Geometry: final body of the model. Coordinates: model frame, mm. Round coordinates to 2 decimals unless told otherwise and drop trailing zeros. Write each loop counter-clockwise with the first axis right and the second up, starting at its lowest first coordinate (ties: lowest second). Pieces come first, ordered by that corner, then holes. Notation, with made-up numbers: (27.25, 21) - (85.25, 21) arc R22 ccw to (85.25, 59) - close; hole circle Ø4 at (28.5, 14). An arc over 180 degrees is marked (long way). Use a Markdown table: item, result. Add a question column.
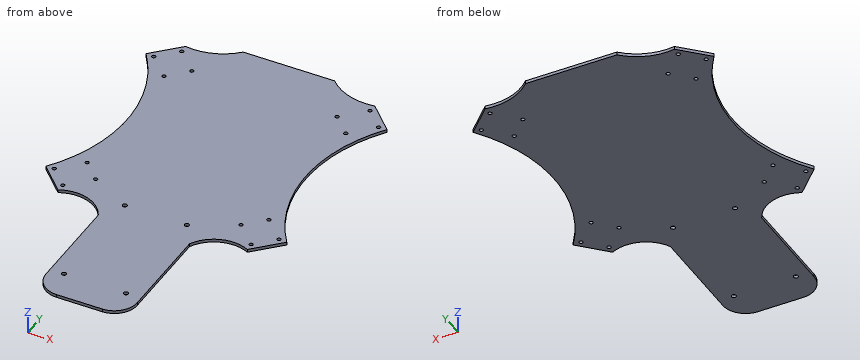
```python
from build123d import *

# Parameters (mm, degrees)
BOSS_EXTRUDE1_DEPTH = 2
SKETCH3_R           = 1.25
CUT_EXTRUDE1_DEPTH  = 188.552659272
SKETCH4_R           = 1.5
CUT_EXTRUDE2_DEPTH  = 188.552659272


with BuildPart() as part:
    # Sketch2 → Boss-Extrude1 (new body)
    with BuildSketch(Plane.XY):
        with BuildLine():
            Line((-79.195959493, 62.225396744), (-62.225396744, 79.195959493))
            ThreePointArc((-62.225396744, 79.195959493), (-44.806778225, 80.702789346), (-30, 90))
            Line((-30, 90), (30, 90))
            ThreePointArc((30, 90), (44.806778225, 80.702789346), (62.225396744, 79.195959493))
            Line((62.225396744, 79.195959493), (79.195959493, 62.225396744))
            ThreePointArc((79.195959493, 62.225396744), (58.781303002, 0), (79.195959493, -62.225396744))
            Line((79.195959493, -62.225396744), (62.225396744, -79.195959493))
            ThreePointArc((62.225396744, -79.195959493), (43.875108319, -77.923881554), (30, -90))
            Line((30, -90), (30, -155))
            ThreePointArc((30, -155), (25.606601718, -165.606601718), (15, -170))
            Line((15, -170), (-15, -170))
            ThreePointArc((-15, -170), (-25.606601718, -165.606601718), (-30, -155))
            Line((-30, -155), (-30, -90))
            ThreePointArc((-30, -90), (-43.875108319, -77.923881554), (-62.225396744, -79.195959493))
            Line((-62.225396744, -79.195959493), (-79.195959493, -62.225396744))
            ThreePointArc((-79.195959493, -62.225396744), (-58.781303002, 0), (-79.195959493, 62.225396744))
        make_face()
    extrude(amount=BOSS_EXTRUDE1_DEPTH)

    # Sketch3 → Cut-Extrude1 (cut, through all)
    with BuildSketch(Plane.XY.offset(2)):
        with Locations((-73.892658634, 61.871843354)):
            Circle(SKETCH3_R)
        with Locations((-59.75052301, 47.72970773)):
            Circle(SKETCH3_R)
        with Locations(Location((-61.871843354, 73.892658634, 0), (0, 0, 180))):
            Circle(SKETCH3_R)
        with Locations(Location((-47.72970773, 59.75052301, 0), (0, 0, 180))):
            Circle(SKETCH3_R)
        with Locations(Location((59.75052301, 47.72970773, 0), (0, 0, 180))):
            Circle(SKETCH3_R)
        with Locations(Location((73.892658634, 61.871843354, 0), (0, 0, 180))):
            Circle(SKETCH3_R)
        with Locations((61.871843354, 73.892658634)):
            Circle(SKETCH3_R)
        with Locations((47.72970773, 59.75052301)):
            Circle(SKETCH3_R)
        with Locations(Location((-59.75052301, -47.72970773, 0), (0, 0, 180))):
            Circle(SKETCH3_R)
        with Locations((-47.72970773, -59.75052301)):
            Circle(SKETCH3_R)
        with Locations((-61.871843354, -73.892658634)):
            Circle(SKETCH3_R)
        with Locations(Location((-73.892658634, -61.871843354, 0), (0, 0, 180))):
            Circle(SKETCH3_R)
        with Locations((59.75052301, -47.72970773)):
            Circle(SKETCH3_R)
        with Locations((73.892658634, -61.871843354)):
            Circle(SKETCH3_R)
        with Locations(Location((61.871843354, -73.892658634, 0), (0, 0, 180))):
            Circle(SKETCH3_R)
        with Locations(Location((47.72970773, -59.75052301, 0), (0, 0, 180))):
            Circle(SKETCH3_R)
    extrude(amount=-CUT_EXTRUDE1_DEPTH, mode=Mode.SUBTRACT)

    # Sketch4 → Cut-Extrude2 (cut, through all)
    with BuildSketch(Plane.XY.offset(2)):
        with Locations((-20.76, -150)):
            Circle(SKETCH4_R)
        with Locations((20, -150)):
            Circle(SKETCH4_R)
        with Locations((-20.76, -74.5)):
            Circle(SKETCH4_R)
        with Locations((20, -74.5)):
            Circle(SKETCH4_R)
    extrude(amount=-CUT_EXTRUDE2_DEPTH, mode=Mode.SUBTRACT)


solid = part.part
```
1) Section C-C, the plane z = 1.6. State how many separate pieces and enclosed holes the cut face has, then the cut area to 3 significant figures.
2) Section D-D, the plane x = 66. Return the cut outline in (y, z), then the cut area to 3 significant figures.
3) Material intervals for L1, parallel to X at y = -150, z = 0.9; L2, parallel to X at y = -74, z = 0.9; L3, parallel to X at y = -139.5, z = 1.9, sorted ascending. Write a range as from..to.
4) Pin query (flat end, axial travel): P1, Ø0.6, axis at y = -112, z = 0.5, coming from the +X side; P2, Ø1, axis at y = -66, z = 0.5, coming from the +X side; P3, Ø1, axis at y = 38.5, z = 1.5, coming from the +X side. Return the tip coordinate at first contact, or that it passes through.
5) Section B-B, the plane y = -99.5. Return the cut outline in (x, z), then the cut area to 3 significant figures.
6) Section A-A, the plane x = -68. Return the cut outline in (y, z).
Output values:
| question | item | result |
|---|---|---|
| 1 | separate pieces | 1 |
| 1 | enclosed holes | 20 |
| 1 | area | 27,100 mm^2 |
| 2 | outline | (-75.42, 0) - (-38.27, 0) - (-38.27, 2) - (-75.42, 2) - close; (38.27, 0) - (75.42, 0) - (75.42, 2) - (38.27, 2) - close |
| 2 | area | 149 mm^2 |
| 3 | L1 | x = -30..-22.26, -19.26..18.5, 21.5..30 |
| 3 | L2 | x = -67.42..-63.12, -60.63..-22.17, -19.35..18.59, 21.41..60.63, 63.12..67.42 |
| 3 | L3 | x = -30..30 |
| 4 | P1 | stops at x = 30 |
| 4 | P2 | stops at x = 75.92 |
| 4 | P3 | stops at x = 66.29 |
| 5 | outline | (-30, 0) - (30, 0) - (30, 2) - (-30, 2) - close |
| 5 | area | 120 mm^2 |
| 6 | outline | (-73.42, 0) - (-43.03, 0) - (-43.03, 2) - (-73.42, 2) - close; (43.03, 0) - (73.42, 0) - (73.42, 2) - (43.03, 2) - close |
